Source: CAD feature listing. Evaluate the final solid. Frame: model axes, mm. Give positions to 0.01 mm unless a question says otherwise; leave off trailing zeros. Write each loop counter-clockwise with the first axis right and the second up, starting at its lowest first coordinate (ties: lowest second). Pieces come first, ordered by that corner, then holes.
```python
from build123d import *

# Parameters (mm, degrees)
SKETCH1_W           = 49
SKETCH1_H           = 19
BOSS_EXTRUDE1_DEPTH = 1.9
SKETCH2_R           = 1.4732
BOSS_EXTRUDE2_DEPTH = 1.9


with BuildPart() as part:
    # Sketch1 → Boss-Extrude1 (new body)
    with BuildSketch(Plane(origin=(0, 0, 0), x_dir=(1, 0, 0), z_dir=(0, 1, 0))):
        Rectangle(SKETCH1_W, SKETCH1_H)
    extrude(amount=BOSS_EXTRUDE1_DEPTH)

    # Sketch2 → Boss-Extrude2 (add)
    # profile 1 of 2: a face of its own
    with BuildSketch(Plane(origin=(0, 0, 0), x_dir=(1, 0, 0), z_dir=(0, 1, 0))):
        with BuildLine():
            Line((-4.75, 14), (-4.75, 9.5))
            Line((-4.75, 9.5), (4.75, 9.5))
            Line((4.75, 9.5), (4.75, 14))
            ThreePointArc((4.75, 14), (0, 18.75), (-4.75, 14))
        make_face()
        with Locations(Location((0, 14, 0), (0, 0, 90))):
            Circle(SKETCH2_R, mode=Mode.SUBTRACT)
    # profile 2 of 2: a face of its own
    with BuildSketch(Plane(origin=(0, 0, 0), x_dir=(1, 0, 0), z_dir=(0, 1, 0))):
        with BuildLine():
            Line((4.75, -14), (4.75, -9.5))
            Line((4.75, -9.5), (-4.75, -9.5))
            Line((-4.75, -9.5), (-4.75, -14))
            ThreePointArc((-4.75, -14), (0, -18.75), (4.75, -14))
        make_face()
        with Locations(Location((0, -14, 0), (0, 0, 90))):
            Circle(SKETCH2_R, mode=Mode.SUBTRACT)
    extrude(amount=BOSS_EXTRUDE2_DEPTH)


solid = part.part
```
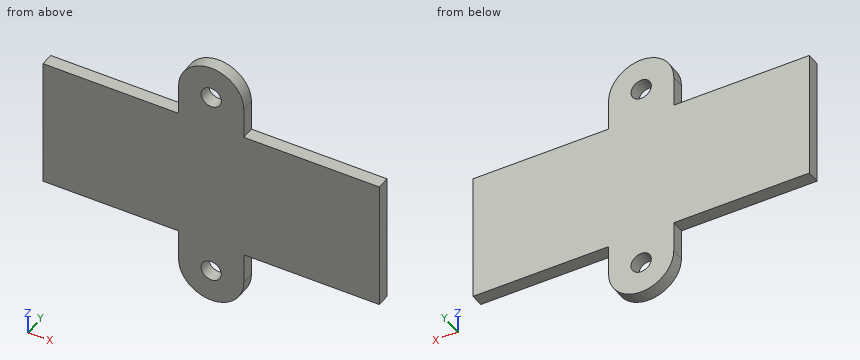
1. Contact query for flat-ended pins moving along their axis: P1, Ø1, axis at y = 1.5, z = 12.5, coming from the -X side; P2, Ø1, axis at y = 1, z = 10.5, coming from the +X side; P3, Ø1.8, axis at x = 0, z = -14, coming from the -Y side. Output: stop coordinate, or through.
2. Cut plane A-A, the plane y = 1.45. Return the cut outline in (x, z).
3. Cut plane D-D, the plane z = -16. Return the cut outline in (x, y), then the cut area to 3 significant figures.
4. Line query: L1, parallel to X at y = 1.5, z = -14; L2, parallel to Z at x = 11, y = 1.35; L3, parallel to Z at x = 0.5, y = 0.3. Output: solid intervals per line, ascending.
5. Cut plane B-B, the plane x = 0. Return the cut outline in (y, z), then the cut area to 3 significant figures.
6. Cut plane C-C, the plane x = 18. Return the cut outline in (y, z), then the cut area to 3 significant figures.
Response values:
1. P1: stops at x = -4.75
1. P2: stops at x = 4.75
1. P3: passes through
2. outline: (-24.5, -9.5) - (-4.75, -9.5) - (-4.75, -14) arc R4.75 ccw to (4.75, -14) - (4.75, -9.5) - (24.5, -9.5) - (24.5, 9.5) - (4.75, 9.5) - (4.75, 14) arc R4.75 ccw to (-4.75, 14) - (-4.75, 9.5) - (-24.5, 9.5) - close; hole circle Ø2.95 at (0, -14); hole circle Ø2.95 at (0, 14)
3. outline: (-4.31, 0) - (4.31, 0) - (4.31, 1.9) - (-4.31, 1.9) - close
3. area: 16.4 mm2
4. L1: x = -4.75 to -1.47, 1.47 to 4.75
4. L2: z = -9.5 to 9.5
4. L3: z = -18.72 to -15.39, -12.61 to 12.61, 15.39 to 18.72
5. outline: (0, -18.75) - (1.9, -18.75) - (1.9, -15.47) - (0, -15.47) - close; (0, -12.53) - (1.9, -12.53) - (1.9, 12.53) - (0, 12.53) - close; (0, 15.47) - (1.9, 15.47) - (1.9, 18.75) - (0, 18.75) - close
5. area: 60.1 mm2
6. outline: (0, -9.5) - (1.9, -9.5) - (1.9, 9.5) - (0, 9.5) - close
6. area: 36.1 mm2
